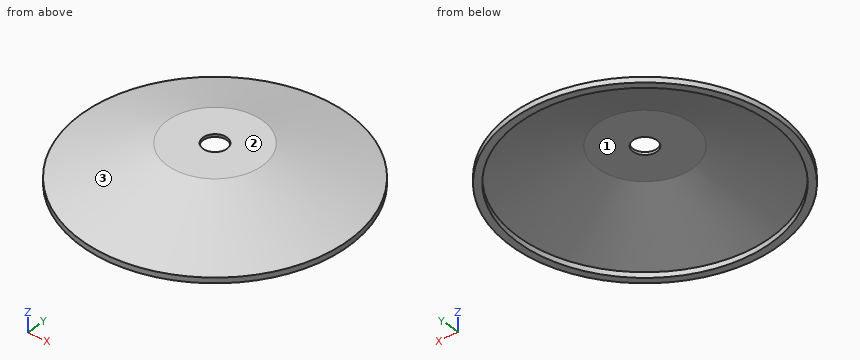
from build123d import *

# Parameters (mm, degrees)
F3_D = 8.8


with BuildPart() as f1:
    # F0 (on Right) → F1 (revolve)
    with BuildSketch(Plane.YZ):
        Polygon((46.5, 2), (46.5, 0), (49.1363636364, 0), (49.1363636364, 2), (17.5, 14), (0, 14), (0, 13), (17.5, 13), align=None)
    revolve(axis=Axis((0, 0, 13.5), (0, 0, -1)))

    # F3 (through all)
    with Locations(Plane.XY.offset(14)):
        with Locations((0, 0)):
            Hole(F3_D / 2)


solid = f1.part
Source: CAD feature listing. Evaluate the final solid. Frame: model axes, mm. Face numbers are marked on the shaded views. Give positions to 0.01 mm unless a question says otherwise; leave off trailing zeros. Write each loop counter-clockwise with the first axis right and the second up, starting at its lowest first coordinate (ties: lowest second). Pieces come first, ordered by that corner, then holes. Notation, with made-up numbers: M 79,77 L 86,77 A12 cw 86,88 Z; hole C 19.25,77 d9. An arc over 180 degrees is marked long. Answer as a JSON object with one key per item and string values.
Q1. Cut plane D-D, the plane z = 6.25. Return the cut outline in (x, y).
Geometry check:
{"outline": "C 0,0 d75.86; hole C 0,0 d70.59"}
Q2. Mould query, pull axis X, two halves, no side actions, for the marked faces 1, 2 and 3. Classes: +X half, -X half, draft (parallel to the pull), parting line (faces both ways), or undercut.
Geometry check:
{"face 1": "undercut", "face 2": "draft", "face 3": "parting line"}
Q3. Ray query, line 1 along X through (y, z) = (0, 0.7); line 2 along Z through (x, y) = (-9.5, 6.5); line 3 along Z through (x, y) = (-16, 35). Return the intervals inside material, ascending.
Geometry check:
{"line 1": "x = -49.14 to -46.5, 46.5 to 49.14", "line 2": "z = 13 to 14", "line 3": "z = 5.04 to 6.04"}
Q4. Contact query for flat-ended pins moving along their axis: P1, Ø6, axis at x = -32.5, y = 18.5, coming from the -Z side; P2, Ø2, axis at x = -7.5, y = -24.5, coming from the +Z side; P3, Ø2, axis at x = -28.5, z = 1.5, coming from the +Y side. Output: stop coordinate, or through.
Geometry check:
{"P1": "stops at z = 4.32", "P2": "stops at z = 11.3", "P3": "stops at y = 40.72"}
Q5. Cut plane C-C, the plane z = 11.75. Return the cut outline in (x, y).
Geometry check:
{"outline": "C 0,0 d46.86; hole C 0,0 d41.59"}
Q6. Cut plane A-A, the plane x = 0. Return the cut outline in (y, z), then the cut area to 3 significant figures.
Geometry check:
{"outline": "M -49.14,0 L -46.5,0 L -46.5,2 L -17.5,13 L -4.4,13 L -4.4,14 L -17.5,14 L -49.14,2 Z; M 4.4,13 L 17.5,13 L 46.5,2 L 46.5,0 L 49.14,0 L 49.14,2 L 17.5,14 L 4.4,14 Z", "area": "97.4 mm^2"}
